Here's how the part is built. I have some questions about the finished solid (model axes, mm). Face numbers are marked on the shaded views. A direction names the side the tool comes from. Give positions to 0.01 mm unless a question says otherwise; leave off trailing zeros. Loops run counter-clockwise (first coordinate to the right, second up) from the corner with the lowest first, then second, coordinate; pieces in that order, holes last.
Q1. Thinking about a two-plate mould opening in Z: for the marked faces 3, 4 and 5, which applies, pulls with the +Z half, pulls with the -Z half, needs draft (parallel to the pull), parting line crosses it, or undercut?
Q2. Suppose I cut it at C-C (y = 0). List the corners of the cut face in (x, z) for me, and give its area (3 significant figures).
Q3. For the marked faces 1 and 2, which set-ups out of +Z, -Z, +X, -X, +Y, -Y let a thin tool reach every point of the face, with its end or its side?
Q4. Suppose I cut it at B-B (x = 0). List the corners of the cut face in (y, z) for me.
Q5. Suppose I cut it at A-A (z = 13.5). List the corners of the cut face in (x, y) for me.
Q6. Suppose I cut it at D-D (x = -9). List the corners of the cut face in (y, z) for me.
Q7. I'm going to push flat-ended pins straight in: P1, Ø5, axis at x = -14, y = -5, coming from the -Z side; P2, Ø1.2, axis at x = 20.5, y = -17, coming from the +Z side; P3, Ø6, axis at x = 7, y = 7.5, coming from the +Z side; P4, Ø1.8, axis at x = 0.5, z = 45, coming from the +Y side. Where does each tip first touch, or does it pass through?
Q8. I need wall thicknesses on probe 1 along Z at (x, y) = (19.5, -15.5); probe 2 along Z at (x, y) = (-4.5, 8); probe 3 along Z at (x, y) = (13, -7.5). Which ranges of each line are inside material? Lowest first, please.
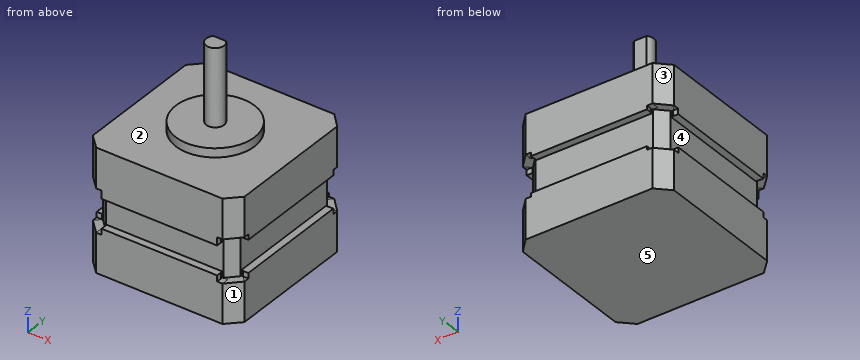
```python
from build123d import *

# Parameters (mm, degrees)
BOSS_EXTRUDE1_DEPTH = 34
SKETCH2_R           = 11
BOSS_EXTRUDE2_DEPTH = 2.5
SKETCH3_R           = 2.5
BOSS_EXTRUDE3_DEPTH = 21.5
CUT_EXTRUDE3_DEPTH  = 2
CUT_EXTRUDE4_DEPTH  = 2
CUT_EXTRUDE5_DEPTH  = 2.3
CUT_EXTRUDE6_DEPTH  = 2.3
CUT_EXTRUDE7_DEPTH  = 2
CUT_EXTRUDE9_DEPTH  = 2
CUT_EXTRUDE10_DEPTH = 2.3
CUT_EXTRUDE11_DEPTH = 2.3
CUT_EXTRUDE12_START = -21.5
CUT_EXTRUDE12_DEPTH = 21.5


with BuildPart() as part:
    # Sketch1 → Boss-Extrude1 (new body)
    with BuildSketch(Plane.XY):
        Polygon((-17.614466094, 21.264089132), (-21.15, 17.728555226), (-21.15, -17.899022103), (-17.614466094, -21.434556009), (17.699167724, -21.434556009), (21.23470163, -17.899022103), (21.23470163, 17.639412218), (17.790617242, 21.264089132), align=None)
    extrude(amount=BOSS_EXTRUDE1_DEPTH)

    # Sketch2 → Boss-Extrude2 (add)
    with BuildSketch(Plane.XY.offset(34)):
        Circle(SKETCH2_R)
    extrude(amount=BOSS_EXTRUDE2_DEPTH)

    # Sketch3 → Boss-Extrude3 (add)
    with BuildSketch(Plane.XY.offset(36.5)):
        Circle(SKETCH3_R)
    extrude(amount=BOSS_EXTRUDE3_DEPTH)

    # Sketch7 → Cut-Extrude3 (cut)
    with BuildSketch(Plane(origin=(21.23470163, 0, 0), x_dir=(0, 0, -1), z_dir=(1, 0, 0))):
        Polygon((-22.997396737, 17.681766019), (-10.997396737, 17.639412218), (-10.997396737, 16.139412218), (-12.497396737, 16.139412218), (-12.497396737, -16.399022103), (-10.997396737, -16.399022103), (-10.997396737, -17.899022103), (-22.997396737, -17.899022103), (-22.997396737, -16.399022103), (-21.497396737, -16.399022103), (-21.497396737, 16.181766019), (-22.997396737, 16.181766019), align=None)
    extrude(amount=-CUT_EXTRUDE3_DEPTH, mode=Mode.SUBTRACT)

    # Sketch6 → Cut-Extrude4 (cut)
    with BuildSketch(Plane(origin=(0, 21.264089132, 0), x_dir=(1, 0, 0), z_dir=(0, 1, 0))):
        Polygon((-17.614466094, -11.039491966), (-17.614466094, -23.039491966), (-16.114466094, -23.039491966), (-16.114466094, -22.039491966), (16.290617242, -22.039491966), (16.290617242, -23.039491966), (17.790617242, -23.039491966), (17.790617242, -11.039491966), (16.290617242, -11.039491966), (16.290617242, -12.039491966), (-16.114466094, -12.039491966), (-16.114466094, -11.039491966), align=None)
    extrude(amount=-CUT_EXTRUDE4_DEPTH, mode=Mode.SUBTRACT)

    # Sketch8 → Cut-Extrude5 (cut)
    with BuildSketch(Plane(origin=(19.96770094, 18.97284881, 0), x_dir=(0, 0, -1), z_dir=(0.724935382761137, 0.6888168775668638, 0))):
        Polygon((-23.039491966, 3.160613175), (-22.997396737, -1.780962582), (-10.997396737, -1.839386825), (-11.039491966, 3.160613175), align=None)
    extrude(amount=-CUT_EXTRUDE5_DEPTH, mode=Mode.SUBTRACT)

    # Sketch10 → Cut-Extrude6 (cut)
    with BuildSketch(Plane(origin=(19.566861866, -19.566861866, 0), x_dir=(0, 0, -1), z_dir=(0.707106781186553, -0.7071067811865421, 0))):
        Polygon((-22.997396737, 2.358681613), (-22.932662916, -2.641318387), (-10.932662916, -2.641318387), (-10.997396737, 2.358681613), align=None)
    extrude(amount=-CUT_EXTRUDE6_DEPTH, mode=Mode.SUBTRACT)

    # Sketch9 → Cut-Extrude7 (cut)
    with BuildSketch(Plane.XZ.offset(21.434556009)):
        Polygon((17.699167724, 22.932662916), (17.699167724, 10.932662916), (16.199167724, 10.932662916), (16.199167724, 12.580798856), (-16.114466094, 12.580798856), (-16.114466094, 10.932662916), (-17.614466094, 10.932662916), (-17.614466094, 22.932662916), (-16.114466094, 22.932662916), (-16.114466094, 20.686804388), (16.199167724, 20.686804388), (16.199167724, 22.932662916), align=None)
    extrude(amount=-CUT_EXTRUDE7_DEPTH, mode=Mode.SUBTRACT)

    # Sketch13 → Cut-Extrude9 (cut)
    with BuildSketch(Plane.ZY.offset(21.15)):
        Polygon((22.997396737, 17.639412218), (10.997396737, 17.639412218), (10.997396737, 16.139412218), (12.497396737, 16.139412218), (12.497396737, -16.399022103), (10.997396737, -16.399022103), (10.997396737, -17.899022103), (22.997396737, -17.899022103), (22.997396737, -16.399022103), (21.497396737, -16.399022103), (21.497396737, 16.181766019), (22.997396737, 16.181766019), align=None)
    extrude(amount=-CUT_EXTRUDE9_DEPTH, mode=Mode.SUBTRACT)

    # Sketch14 → Cut-Extrude10 (cut)
    with BuildSketch(Plane(origin=(-19.439277613, 19.439277613, 0), x_dir=(0, 0, 1), z_dir=(-0.707106781186543, 0.7071067811865521, 0))):
        Polygon((11.039491966, 2.580673199), (10.997396737, -2.482360427), (22.997396737, -2.482360427), (23.039491966, 2.580673199), align=None)
    extrude(amount=-CUT_EXTRUDE10_DEPTH, mode=Mode.SUBTRACT)

    # Sketch15 → Cut-Extrude11 (cut)
    with BuildSketch(Plane(origin=(-19.524511051, -19.524511051, 0), x_dir=(0, 0, 1), z_dir=(-0.7071067811865381, -0.707106781186557, 0))):
        Polygon((10.997396737, 2.298788516), (10.932662916, -2.701211484), (22.932662916, -2.701211484), (22.997396737, 2.298788516), align=None)
    extrude(amount=-CUT_EXTRUDE11_DEPTH, mode=Mode.SUBTRACT)

    # Sketch16 → Cut-Extrude12 (cut)
    with BuildSketch(Plane.XY.offset(58).offset(CUT_EXTRUDE12_START)):
        with BuildLine():
            Line((-1.764671013, 1.770857481), (1.764671013, 1.770857481))
            ThreePointArc((1.764671013, 1.770857481), (0, 2.5), (-1.764671013, 1.770857481))
        make_face()
    extrude(amount=CUT_EXTRUDE12_DEPTH, mode=Mode.SUBTRACT)


solid = part.part
```
Solutions:
1. face 3: needs draft
1. face 4: undercut
1. face 5: pulls with the -Z half
2. outline: (-21.15, 0) - (21.23, 0) - (21.23, 12.5) - (19.23, 12.5) - (19.23, 21.5) - (21.23, 21.5) - (21.23, 34) - (11, 34) - (11, 36.5) - (2.5, 36.5) - (2.5, 58) - (-2.5, 58) - (-2.5, 36.5) - (-11, 36.5) - (-11, 34) - (-21.15, 34) - (-21.15, 21.5) - (-19.15, 21.5) - (-19.15, 12.5) - (-21.15, 12.5) - close
2. area: 1,570 mm2
3. face 1: +Z, -Z, +X, -Y
3. face 2: +Z
4. outline: (-21.43, 0) - (21.26, 0) - (21.26, 12.04) - (19.26, 12.04) - (19.26, 22.04) - (21.26, 22.04) - (21.26, 34) - (11, 34) - (11, 36.5) - (1.77, 36.5) - (1.77, 58) - (-2.5, 58) - (-2.5, 36.5) - (-11, 36.5) - (-11, 34) - (-21.43, 34) - (-21.43, 20.69) - (-19.43, 20.69) - (-19.43, 12.58) - (-21.43, 12.58) - close
5. outline: (-19.15, -16.65) - (-16.36, -19.43) - (16.45, -19.43) - (19.23, -16.65) - (19.23, 16.41) - (16.52, 19.26) - (-16.36, 19.26) - (-19.15, 16.48) - close
6. outline: (-21.43, 0) - (21.26, 0) - (21.26, 12.04) - (19.26, 12.04) - (19.26, 22.04) - (21.26, 22.04) - (21.26, 34) - (6.32, 34) - (6.32, 36.5) - (-6.32, 36.5) - (-6.32, 34) - (-21.43, 34) - (-21.43, 20.69) - (-19.43, 20.69) - (-19.43, 12.58) - (-21.43, 12.58) - close
7. P1: stops at z = 0
7. P2: stops at z = 34
7. P3: stops at z = 36.5
7. P4: stops at y = 1.77
8. probe 1: z = 0 to 12.5, 21.5 to 34
8. probe 2: z = 0 to 36.5
8. probe 3: z = 0 to 34
